Could you check a few things on this drawing? It's one solid part, dimensions in mm from its lowest x, y, z. A direction names the side the tool comes from. Give positions to 0.01 mm unless a question says otherwise; leave off trailing zeros. Order: outer loops, then holes, each group sorted by start corner. A loop starts at its lowest first (then second) coordinate and runs counter-clockwise, first axis right, second up. Notation, with made-up numbers: (31.5, 29.25) -> (41.5, 29.25) arc R23 ccw to (41.5, 68.25) -> close; hole circle Ø11 at (28, 60). An arc over 180 degrees is marked (long way). Answer as a JSON object with one key per item and string values.
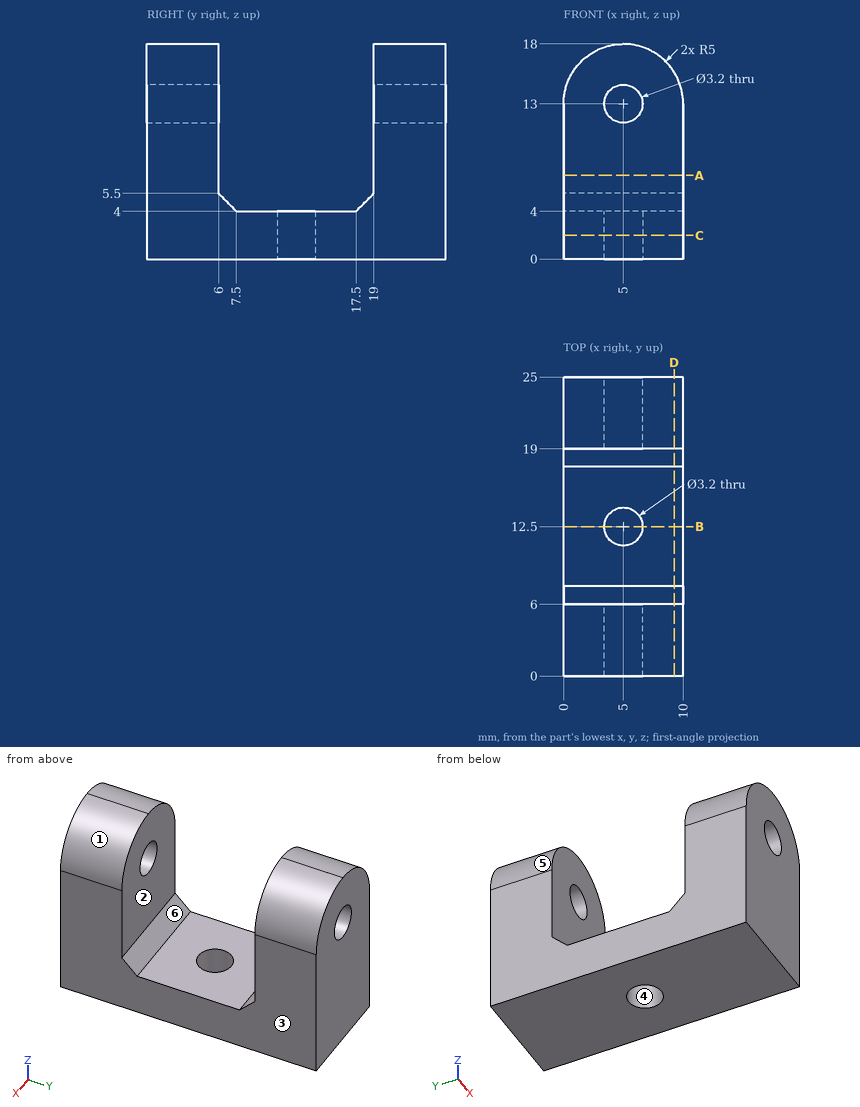
1. Please list where these lines run through material, in increasing order: L1, parallel to Y at x = 1, z = 15; L2, parallel to X at y = 21.9, z = 13; L3, parallel to Z at x = 4.75, y = 8.
Worked answers:
{"L1": "0 to 6, 19 to 25", "L2": "0 to 3.4, 6.6 to 10", "L3": "0 to 4"}
2. If we section it at B-B on y = 12.5: Please give me the cut outline in (x, z).
Worked answers:
{"outline": "(0, 0) -> (3.4, 0) -> (3.4, 4) -> (0, 4) -> close; (6.6, 0) -> (10, 0) -> (10, 4) -> (6.6, 4) -> close"}
3. If we section it at C-C on z = 2: Please give me the cut outline in (x, y).
Worked answers:
{"outline": "(0, 0) -> (10, 0) -> (10, 25) -> (0, 25) -> close; hole circle Ø3.2 at (5, 12.5)"}
4. If we section it at D-D on x = 9.25: Please give me the cut outline in (y, z).
Worked answers:
{"outline": "(0, 0) -> (25, 0) -> (25, 15.63) -> (19, 15.63) -> (19, 5.5) -> (17.5, 4) -> (7.5, 4) -> (6, 5.5) -> (6, 15.63) -> (0, 15.63) -> close"}
5. For the marked faces 1 and 2, which set-ups out of +Z, -Z, +X, -X, +Y, -Y let a thin tool reach every point of the face, with its end or its side?
Worked answers:
{"face 1": "+Z, +X, +Y, -Y", "face 2": "+Z, +X, -X"}
6. Will this pin go through, and if not, where does the flat tip stop? pin 1 Ø1.9 at (x, z) = (5, 13) entering from +Y.
Worked answers:
{"pin 1": "through"}
7. If we mould it in two halves opening along X, with no side actions, what happens to the marked faces 3, 4, 5 and 6? For each: +X half, -X half, draft (parallel to the pull), parting line (faces both ways), or undercut.
Worked answers:
{"face 3": "+X half", "face 4": "undercut", "face 5": "-X half", "face 6": "draft"}
8. If we section it at A-A on z = 7: Please give me the cut outline in (x, y).
Worked answers:
{"outline": "(0, 0) -> (10, 0) -> (10, 6) -> (0, 6) -> close; (0, 19) -> (10, 19) -> (10, 25) -> (0, 25) -> close"}
